from build123d import *

# Parameters (mm, degrees)
BOSS_EXTRUDE1_START = -7.151569
BOSS_EXTRUDE1_DEPTH = 14.303137569
CAVITY3_START       = -3.125287666
CAVITY3_DEPTH       = 9.3420001
CAVITY3_START_2     = -7.554089613
CAVITY3_2_OUTLINE_R = 3.278779553
CAVITY3_2_DEPTH     = 2.904801847
CAVITY3_START_3     = 0.374712334
CAVITY3_3_DEPTH     = 2.960969152
CAVITY3_START_4     = -3.175
CAVITY3_4_DEPTH     = 6.35


with BuildPart() as part:
    # Sketch1 → Boss-Extrude1 (new body)
    with BuildSketch(Plane.XY.offset(BOSS_EXTRUDE1_START)):
        Polygon((-10, 0), (10.513602901, 0), (-1.192334822, -10.153914519), align=None)
    extrude(amount=BOSS_EXTRUDE1_DEPTH)

    # Cavity3: read off the stored shape, not the designer's step
    # Cavity3 outline → Cavity3 (cut)
    with BuildSketch(Plane(origin=(0, 0, 0), x_dir=(0.6552536158947596, -0.7554089613294528, 0), z_dir=(0.7554089613294528, 0.6552536158947598, 0)).offset(CAVITY3_START)):
        with BuildLine():
            Line((3.079076317, -3.175), (3.079076317, 3.175))
            Line((3.079076317, 3.175), (-0.989318671, 3.175))
            ThreePointArc((-0.989318671, 3.175), (-3.449703236, 0), (-0.989318671, -3.175))
            Line((-0.989318671, -3.175), (3.079076317, -3.175))
        make_face()
    extrude(amount=CAVITY3_DEPTH, mode=Mode.SUBTRACT)

    # Cavity3 2 outline → Cavity3 2 (cut)
    with BuildSketch(Plane(origin=(0, 0, 0), x_dir=(0.6552536158947596, -0.7554089613294528, 0), z_dir=(0.7554089613294528, 0.6552536158947598, 0)).offset(CAVITY3_START_2)):
        with Locations((-0.170923683, 0)):
            Circle(CAVITY3_2_OUTLINE_R)
    extrude(amount=CAVITY3_2_DEPTH, mode=Mode.SUBTRACT)

    # Cavity3 3 outline → Cavity3 3 (cut)
    with BuildSketch(Plane(origin=(0, 0, 0), x_dir=(0.6552536158947596, -0.7554089613294528, 0), z_dir=(0.7554089613294528, 0.6552536158947598, 0)).offset(CAVITY3_START_3)):
        with BuildLine():
            Line((3.079076317, 0.433468981), (3.079076317, -0.433468981))
            ThreePointArc((3.079076317, -0.433468981), (3.10785587, 0), (3.079076317, 0.433468981))
        make_face()
    extrude(amount=CAVITY3_3_DEPTH, mode=Mode.SUBTRACT)

    # Cavity3 4 outline → Cavity3 4 (cut)
    with BuildSketch(Plane.XY.offset(CAVITY3_START_4)):
        Polygon((-0.343294419, -4.373817886), (4.699060398, 0), (-4.137212856, 0), align=None)
    extrude(amount=CAVITY3_4_DEPTH, mode=Mode.SUBTRACT)

    # Cavity3 5: loft between two sections, ruled curve by curve
    cavity3_5_from = [
        Edge.make_three_point_arc((2.300636945, -2.08043023, -3.175), (4.699060398, 0, 0), (2.300636945, -2.08043023, 3.175)),
        Edge.make_three_point_arc((2.300636945, -2.08043023, 3.175), (-0.097786507, -4.160860461, 0), (2.300636945, -2.08043023, -3.175)),
    ]
    cavity3_5_to = [
        Edge.make_three_point_arc((4.797153222, -4.958538373, -5.842), (9.210252374, -1.130546749, 0), (4.797153222, -4.958538373, 5.842)),
        Edge.make_three_point_arc((4.797153222, -4.958538373, 5.842), (0.38405407, -8.786529997, 0), (4.797153222, -4.958538373, -5.842)),
    ]
    cavity3_5 = Solid(Shell([*[Face.make_surface_from_curves(cavity3_5_from[k], cavity3_5_to[k]) for k in range(2)], Face(Wire(cavity3_5_from)), Face(Wire(cavity3_5_to))]))
    add(cavity3_5, mode=Mode.SUBTRACT)

    # Cavity3 6: loft between two sections, ruled curve by curve
    cavity3_6_from = [
        Edge.make_three_point_arc((-3.643299316, -2.933988714, -3.304179553), (-1.478223716, -5.429995558, 0), (-3.643299316, -2.933988714, 3.304179553)),
        Edge.make_three_point_arc((-3.643299316, -2.933988714, 3.304179553), (-5.808374915, -0.43798187, 0), (-3.643299316, -2.933988714, -3.304179553)),
    ]
    cavity3_6_to = [
        Edge.make_three_point_arc((-5.81842535, -4.820727252, -5.075783124), (-2.492500105, -8.655019309, 0), (-5.81842535, -4.820727252, 5.075783124)),
        Edge.make_three_point_arc((-5.81842535, -4.820727252, 5.075783124), (-9.144350595, -0.986435194, 0), (-5.81842535, -4.820727252, -5.075783124)),
    ]
    cavity3_6 = Solid(Shell([*[Face.make_surface_from_curves(cavity3_6_from[k], cavity3_6_to[k]) for k in range(2)], Face(Wire(cavity3_6_from)), Face(Wire(cavity3_6_to))]))
    add(cavity3_6, mode=Mode.SUBTRACT)

    # Cavity3 7: loft between two sections, ruled curve by curve
    cavity3_7_from = [
        Edge.make_three_point_arc((-2.472868671, -1.918738762, -2.54), (-0.808524487, -3.837477524, 0), (-2.472868671, -1.918738762, 2.54)),
        Edge.make_three_point_arc((-2.472868671, -1.918738762, 2.54), (-4.137212855, 0, 0), (-2.472868671, -1.918738762, -2.54)),
    ]
    cavity3_7_to = [
        Edge.make_three_point_arc((-3.624111928, -2.917345272, -3.278779553), (-1.47567977, -5.394164729, 0), (-3.624111928, -2.917345272, 3.278779553)),
        Edge.make_three_point_arc((-3.624111928, -2.917345272, 3.278779553), (-5.772544086, -0.440525816, 0), (-3.624111928, -2.917345272, -3.278779553)),
    ]
    cavity3_7 = Solid(Shell([*[Face.make_surface_from_curves(cavity3_7_from[k], cavity3_7_to[k]) for k in range(2)], Face(Wire(cavity3_7_from)), Face(Wire(cavity3_7_to))]))
    add(cavity3_7, mode=Mode.SUBTRACT)


solid = part.part
Geometry: final body of the model. Coordinates: model frame, mm. A direction names the side the tool comes from. Give positions to 0.01 mm unless a question says otherwise; leave off trailing zeros. Answer as a JSON object with one key per item and string values.
Q1. Access query for faces 1 (the flat face through (4.116, -0.506, 2.536)), 2 (the flat face through (0, -3, 7.152)). Directions: +Z, -Z, +X, -X, +Y, -Y. A direction counts if a zero-diameter tool reaches every point of the face in a straight line with its end or side. Return the directions, or none.
Entries:
{"face 1": "+Y", "face 2": "+Z, +X, -X, +Y, -Y"}
Q2. Section A-A (z = -1.75). State how many separate pieces and enclosed holes the cut face has, plus the area to 3 significant figures.
Entries:
{"separate pieces": "3", "enclosed holes": "0", "area": "24.2 mm^2"}
Q3. Draft query along X for faces 3 (the flat face through (2.1, -7.3, -4.9)), 4 (the flat face through (4.205, -0.429, -2.521)), 5 (the flat face through (-4.556, -6.276, -4.868)), 6 (the flat face through (0, -1, -3.175)). Return one class per face: released by +X, released by -X, zero draft, split by the parting line, or undercut.
Entries:
{"face 3": "released by +X", "face 4": "undercut", "face 5": "released by -X", "face 6": "undercut"}
Q4. First-contact query: pin 1 (3 mm diameter, centred on y = -4, z = 1.5, fed in from +X); pin 2 (1.5 mm diameter, centred on y = -2, z = 2.5, fed in from -X); pin 3 (1 mm diameter, centred on y = -1, z = 0, fed in from -X); pin 4 (1 mm diameter, centred on x = -5.5, y = -7.5, fed in from -Z). Flat tips, straight axial feed; report the tip coordinate or a pass-through.
Entries:
{"pin 1": "stops at x = 1.19", "pin 2": "stops at x = -8.92", "pin 3": "stops at x = -9.57", "pin 4": "passes through"}
Q5. Material intervals for probe 1 along Z at (x, y) = (-0.75, -1.5) (3 decimals); probe 2 along Y at (x, z) = (-6, 2.5); probe 3 along Z at (x, y) = (3.5, -4.5), sorted ascending.
Entries:
{"probe 1": "z = -7.152 to -3.175, 3.175 to 7.152", "probe 2": "y = -1.3 to 0", "probe 3": "z = -7.15 to -4.96, 4.96 to 7.15"}
